```python
from build123d import *

# Parameters (mm, degrees)
BOSS_EXTRUDE1_DEPTH = 6
SKETCH2_R           = 35
BOSS_EXTRUDE2_DEPTH = 15


with BuildPart() as part:
    # Sketch1 → Boss-Extrude1 (new body)
    with BuildSketch(Plane(origin=(0, 0, 0), x_dir=(1, 0, 0), z_dir=(0, 1, 0))):
        with BuildLine():
            Line((-20.075175272, 28.67032155), (110.989151814, 120.442551366))
            ThreePointArc((110.989151814, 120.442551366), (159.734648636, 111.847405088), (151.139502359, 63.101908266))
            Line((151.139502359, 63.101908266), (20.075175272, -28.67032155))
            ThreePointArc((20.075175272, -28.67032155), (-28.67032155, -20.075175272), (-20.075175272, 28.67032155))
        make_face()
    extrude(amount=-BOSS_EXTRUDE1_DEPTH)

    # Sketch2 → Boss-Extrude2 (add)
    with BuildSketch(Plane.XZ.offset(6)):
        Circle(SKETCH2_R)
    extrude(amount=BOSS_EXTRUDE2_DEPTH)


solid = part.part
```
The model under review builds one solid part; all positions refer to its coordinate system, in mm. A direction names the side the tool comes from. Round coordinates to 2 decimals unless told otherwise and drop trailing zeros. Write each loop counter-clockwise with the first axis right and the second up, starting at its lowest first coordinate (ties: lowest second). Pieces come first, ordered by that corner, then holes. Notation, with made-up numbers: (78.5, 40) - (98.5, 40) arc R32 ccw to (98.5, 79) - close; hole circle Ø9 at (-18.75, -17.75). An arc over 180 degrees is marked (long way). Answer as CSV lines item,"result". Start each with the question number.
(1) To check wall thickness, follow line 1 (Y direction, x = 57.5, z = -32); line 2 (X direction, y = -12.5, z = 0); line 3 (Z direction, x = -11, y = -16.75). State the ranges of each line that lie inside material, in increasing order.
(2) We need section D-D on y = -18.75. State the section outline as (x, z) points, plus the area to 3 significant figures.
(3) For pin 1 Ø1.5 at (y, z) = (-4, -109.5) entering from -X; pin 2 Ø12 at (x, y) = (117.5, -6.5) entering from +Z; pin 3 Ø12 at (y, z) = (-6.5, -19.5) entering from +X, all flat-tipped, find the tip position at first contact; note any pin that passes through.
(4) We need section B-B on x = -1. State the section outline as (y, z) points, plus the area to 3 significant figures.
(5) For faces 1 (the cylindrical face through (-25.8, -12.69, 23.65)), 2 (the flat face through (0, -21, 0)), list the 3-axis set-ups (+Z, -Z, +X, -X, +Y, -Y) from which the entire face can be reached by the end or side of a thin tool; tool diameter is ignored.
(6) We need section C-C on z = 0. State the section outline as (x, y) points, plus the area to 3 significant figures.
(7) We need section A-A on y = -2.75. State the section outline as (x, z) points.
Worked answers:
1,line 1,"-6 to 0"
1,line 2,"-35 to 35"
1,line 3,"-33.23 to 33.23"
2,outline,"circle Ø70 at (0, 0)"
2,area,"3,850 mm²"
3,pin 1,"x = 94.29"
3,pin 2,"z = -35.36"
3,pin 3,"x = 97.41"
4,outline,"(-21, -34.99) - (-6, -34.99) - (-6, -42.03) - (0, -42.03) - (0, 34.99) - (-21, 34.99) - close"
4,area,"1,510 mm²"
5,face 1,"-Y"
5,face 2,"+Z, -Z, +X, -X, -Y"
6,outline,"(-35, -21) - (35, -21) - (35, -6) - (61.02, -6) - (61.02, 0) - (-35, 0) - close"
6,area,"1,630 mm²"
7,outline,"(-20.08, -28.67) - (110.99, -120.44) arc R35 ccw to (151.14, -63.1) - (20.08, 28.67) arc R35 ccw to start"
